Autodesk Inventor part; units mm, degrees
ref_plane "YZ Plane" through (0, 0, 0) normal (1, 0, 0) x (0, 1, 0)
ref_plane "XZ Plane" through (0, 0, 0) normal (0, 1, 0) x (-1, 0, 0)
ref_plane "XY Plane" through (0, 0, 0) normal (0, 0, 1) x (1, 0, 0)
sketch "main" plane through (0, 0, 0) normal (0, 0, 1) x (1, 0, 0)
  line L0 (46.0129, -12.1958) -> (-42.8871, -12.1958)
  circle A0 centre (46.0129, -12.1958) radius 5.5563
  arc A1 (45.534, -24.8867) -> (45.5846, 0.497) centre (46.0129, -12.1958) ccw
  line L1 (-46.0418, -15.1681) -> (-39.7426, -15.1681)
  line L2 (-39.7426, -15.1681) -> (-39.7426, -8.8689)
  line L3 (-39.7426, -8.8689) -> (-46.0418, -8.8689)
  line L4 (-46.0418, -8.8689) -> (-46.0418, -15.1681)
  line L5 (-46.0418, -15.1681) -> (-39.7426, -8.8689) construction
  line L6 (-39.7426, -15.1681) -> (-46.0418, -8.8689) construction
  arc A2 (-43.2133, -2.4989) -> (-43.2513, -21.5368) centre (-42.8922, -12.0185) ccw
  line L7 (-43.2133, -2.4989) -> (45.5846, 0.497)
  line L8 (-43.2513, -21.5368) -> (45.534, -24.8867)
  circle A3 centre (12.7, -12.1958) radius 2.1844
  circle A4 centre (0, -12.1958) radius 2.1844
  circle A5 centre (-12.7, -12.1958) radius 2.1844
  point P0 (-14.9546, -14.9924)
  point P1 (-63.2594, -31.7725)
  point P2 (-42.8922, -12.0185)
  dimension "d0" = 88.9
  dimension "d2" = 11.1125
  dimension "d3" = 25.4
  dimension "d4" = 6.2992
  dimension "d5" = 6.2992
  dimension "d6" = 19.05
  dimension "d9" = 4.3688
  dimension "d12" = 12.7
sketch "Sketch1" plane through (0, 0, 0) normal (1, 0, 0) x (0, 1, 0)
  line L0 (0, 0) -> (-0.1504, 88.8999)
  circle A0 centre (0, 0) radius 5.5563
  arc A1 (-12.6918, 0.4574) -> (12.692, 0.4497) centre (0, 0) ccw
  line L1 (-3.128, 92.0495) -> (-3.1174, 85.7503)
  line L2 (-3.1174, 85.7503) -> (3.1818, 85.7609)
  line L3 (3.1818, 85.7609) -> (3.1711, 92.0601)
  line L4 (3.1711, 92.0601) -> (-3.128, 92.0495)
  line L5 (-3.128, 92.0495) -> (3.1818, 85.7609) construction
  line L6 (-3.1174, 85.7503) -> (3.1711, 92.0601) construction
  arc A2 (9.5459, 89.2425) -> (-9.4919, 89.2482) centre (0.0269, 88.9052) ccw
  line L7 (9.5459, 89.2425) -> (12.692, 0.4497)
  line L8 (-9.4919, 89.2482) -> (-12.6918, 0.4574)
  circle A3 centre (-0.0563, 33.3128) radius 2.1844
  circle A4 centre (-0.0778, 46.0128) radius 2.1844
  circle A5 centre (-0.0993, 58.7128) radius 2.1844
  point P0 (0, 0)
extrude "Extrusion1" add sketch "Sketch1" along normal blind 1.5875
properties part number "Gusset" material "Acetal Resin, White"
The model under review builds one solid part; all positions refer to its coordinate system, in mm. Round coordinates to 2 decimals unless told otherwise and drop trailing zeros. Loops run counter-clockwise (first coordinate to the right, second up) from the corner with the lowest first, then second, coordinate; pieces in that order, holes last. Notation, with made-up numbers: M -21,53.5 L 17,53.5 A22 cw 17,90.5 Z; hole C 83.5,57 d8. An arc over 180 degrees is marked long. Put each result on its own line as item: value.
Q1. To check wall thickness, follow L1, parallel to Z at x = 0.85, y = 0; L2, parallel to Y at x = 0.65, z = 0; L3, parallel to Z at x = 1.45, y = -0.5. State the ranges of each line that lie inside material, in increasing order.
Result set:
L1: z = -12.7 to -5.56, 5.56 to 31.13, 35.5 to 43.83, 48.2 to 56.53, 60.89 to 85.76, 92.05 to 98.43
L2: y = -12.7 to -5.56, 5.56 to 12.7
L3: z = -12.69 to -5.53, 5.53 to 31.17, 35.45 to 43.87, 48.16 to 56.57, 60.86 to 85.75, 92.05 to 98.42
Q2. Mouldability with a two-part tool opening along Y and no side actions: class faces 1 (the flat face through (1.588, -0.2, 43.6)), 2 (the cylindrical face through (0.783, 0.282, -12.697)), 3 (the cylindrical face through (0.783, -0.341, 31.147)) as released by +Y, released by -Y, zero draft, split by the parting line, or undercut.
Result set:
face 1: zero draft
face 2: split by the parting line
face 3: undercut
Q3. Consider section A-A, the plane x = 0.6. Give the boundary of the cut face in (y, z).
Result set:
outline: M -12.69,0.46 A12.7 ccw long 12.69,0.45 L 9.55,89.24 A9.52 ccw -9.49,89.25 Z; hole C 0,0 d11.11; hole M -3.13,92.05 L -3.12,85.75 L 3.18,85.76 L 3.17,92.06 Z; hole C -0.1,58.71 d4.37; hole C -0.08,46.01 d4.37; hole C -0.06,33.31 d4.37
Q4. Consider section C-C, the plane z = 30. Give the boundary of the cut face in (x, y), then the cut area to 3 significant figures.
Result set:
outline: M 0,-11.63 L 1.59,-11.63 L 1.59,11.64 L 0,11.64 Z
area: 36.9 mm²
Q5. Consider section B-B, the plane z = 88. Give the boundary of the cut face in (x, y), then the cut area to 3 significant figures.
Result set:
outline: M 0,-9.54 L 1.59,-9.54 L 1.59,-3.12 L 0,-3.12 Z; M 0,3.18 L 1.59,3.18 L 1.59,9.59 L 0,9.59 Z
area: 20.4 mm²
Q6. Consider section D-D, the plane y = 7.75. Give the boundary of the cut face in (x, z).
Result set:
outline: M 0,-10.06 L 1.59,-10.06 L 1.59,94.48 L 0,94.48 Z
Q7. For pin 1 (7 mm diameter, centred on y = -0.06, z = 33.31, fed in from -X); pin 2 (3.5 mm diameter, centred on y = -0.1, z = 58.71, fed in from +X), all flat-tipped, find the tip position at first contact; note any pin that passes through.
Result set:
pin 1: stops at x = 0
pin 2: passes through
